Verification items for the finished model (mm, model axes). A direction names the side the tool comes from. Coordinates: 2 decimals unless noted, no trailing zeros. Write each loop counter-clockwise with the first axis right and the second up, starting at its lowest first coordinate (ties: lowest second). Pieces come first, ordered by that corner, then holes. Notation, with made-up numbers: M -9.75,23.25 L 36.25,23.25 A21 cw 36.25,41.25 Z; hole C 58.25,86.25 d6. An arc over 180 degrees is marked long. Answer in a Markdown table with one row per item.
Autodesk Inventor part; units mm, degrees
ref_plane "YZ Plane" through (0, 0, 0) normal (1, 0, 0) x (0, 1, 0)
ref_plane "XZ Plane" through (0, 0, 0) normal (0, 1, 0) x (-1, 0, 0)
ref_plane "XY Plane" through (0, 0, 0) normal (0, 0, 1) x (1, 0, 0)
sketch "Sketch1" plane through (0, 0, 0) normal (0, 1, 0) x (-1, 0, 0)
  line L0 (-25, 23) -> (25, 23)
  line L1 (25, 23) -> (25, -23)
  line L2 (25, -23) -> (-25, -23)
  line L3 (-25, -23) -> (-25, 23)
  line L4 (-25, 23) -> (25, -23) construction
  line L5 (25, 23) -> (-25, -23) construction
  circle A0 centre (12, 0) radius 4.15
  circle A1 centre (-15, -12) radius 2.65
  line L6 (25, 0) -> (-25, 0) construction
  circle A2 centre (-15, 12) radius 2.65
  point P0 (0, 0)
  dimension "d0" = 46
  dimension "d1" = 50
  dimension "d2" = 23
  dimension "d3" = 13
  dimension "d4" = 8.3
  dimension "d5" = 11
  dimension "d6" = 10
  dimension "d7" = 5.3
extrude "Extrusion1" add sketch "Sketch1" along normal blind 8
sketch "Sketch2" plane through (0, 0, 0) normal (0, -1, 0) x (1, 0, 0)
  line L0 (25, -23) -> (-25, -23)
  line L1 (25, 23) -> (25, -23)
  line L2 (-25, 23) -> (25, 23)
  line L3 (-25, -23) -> (-25, 23)
  circle A0 centre (15, 12) radius 2.65 construction
  circle A1 centre (15, -12) radius 2.65 construction
  circle A2 centre (-12, 0) radius 4.15
  circle A3 centre (15, -12) radius 2.65 construction
  circle A4 centre (15, -12) radius 5
  circle A5 centre (15, 12) radius 5
  point P0 (0, 0)
  dimension "d10" = 10
  dimension "d11" = 10
extrude "Extrusion2" cut sketch "Sketch2" against normal blind 5 contours A4 | A5
sketch "Sketch3" plane through (0, 8, 0) normal (0, 1, 0) x (1, 0, 0)
  circle A0 centre (13.5, 18.5) radius 3.15
  line L0 (25, -23) -> (25, 23)
  line L1 (25, 0) -> (-25, 0) construction
  line L2 (-25, 23) -> (-25, -23)
  line L3 (25, 23) -> (-25, 23)
  circle A1 centre (13.5, -18.5) radius 3.15
  point P0 (0, 0)
  dimension "d14" = 4.5
  dimension "d15" = 11.5
  dimension "d16" = 6.3
extrude "Extrusion3" cut sketch "Sketch3" against normal blind 3
sketch "Sketch5" plane through (0, 0, 0) normal (0, -1, 0) x (1, 0, 0)
  circle A0 centre (-12, 0) radius 4.15
  point P0 (0, 0)
extrude "Extrusion5" add sketch "Sketch5" against normal blind 1
equation "\"d11\" = d10"
properties part number "Linear Rail End Cap"
1) Sectioned sample at B-B (y = 7). Record the cut outline in (x, z), then the cut area to 3 significant figures.
Response values:
| item | result |
|---|---|
| outline | M -25,-23 L 25,-23 L 25,23 L -25,23 Z; hole C -12,0 d8.3; hole C 13.5,-18.5 d6.3; hole C 13.5,18.5 d6.3; hole C 15,-12 d5.3; hole C 15,12 d5.3 |
| area | 2,140 mm² |
2) Sectioned sample at C-C (x = 19). Record the cut outline in (y, z).
Response values:
| item | result |
|---|---|
| outline | M 0,-23 L 8,-23 L 8,23 L 0,23 L 0,15 L 5,15 L 5,9 L 0,9 L 0,-9 L 5,-9 L 5,-15 L 0,-15 Z |
3) Depth check by flat-ended pin: pin 1 (4 mm diameter, centred on x = 15, z = -12, fed in from -Y); pin 2 (6.5 mm diameter, centred on x = -12.5, z = 0, fed in from +Y); pin 3 (5 mm diameter, centred on x = 13.5, z = -11, fed in from -Y); pin 4 (5.5 mm diameter, centred on x = 13.5, z = 18.5, fed in from +Y). Enter the tip coordinate at first touch or a pass-through.
Response values:
| item | result |
|---|---|
| pin 1 | passes through |
| pin 2 | stops at y = 1 |
| pin 3 | stops at y = 5 |
| pin 4 | stops at y = 5 |
4) Release check for a two-part mould opening along X. For faces 1 (the face through (19.77, 2.46, 13.5)), 2 (the face through (0, 4, 23)), 3 (the face through (-25, 4, 0)), 4 (the face through (10.353, 6.521, 18.362)) record: +X half, -X half, draft (parallel to the pull), parting line (faces both ways), or undercut.
Response values:
| item | result |
|---|---|
| face 1 | undercut |
| face 2 | draft |
| face 3 | -X half |
| face 4 | undercut |
5) Sectioned sample at D-D (z = -12). Record the cut outline in (x, y).
Response values:
| item | result |
|---|---|
| outline | M -25,0 L 10,0 L 10,5 L 12.35,5 L 12.35,8 L -25,8 Z; M 17.65,5 L 20,5 L 20,0 L 25,0 L 25,8 L 17.65,8 Z |
6) Sectioned sample at A-A (y = 2). Record the cut outline in (x, z).
Response values:
| item | result |
|---|---|
| outline | M -25,-23 L 25,-23 L 25,23 L -25,23 Z; hole C -12,0 d8.3; hole C 15,-12 d10; hole C 15,12 d10 |
7) Thickness scan on L1, parallel to Z at x = 15, y = 2.7; L2, parallel to X at y = 7, z = -18.5; L3, parallel to X at y = 5.75, z = 0. Record the ranges inside material, lowest first. Write a range as [from, to].
Response values:
| item | result |
|---|---|
| L1 | z = [-23, -17], [-7, 7], [17, 23] |
| L2 | x = [-25, 10.35], [16.65, 25] |
| L3 | x = [-25, -16.15], [-7.85, 25] |
8) Tool access check on faces 5 (the face through (0, 4, -23)), 6 (the face through (17, 5, -10)), 7 (the face through (-12, 1, 0)). Record the directions out of +Z, -Z, +X, -X, +Y, -Y that give a thin tool (end or side, any length) a straight path to the whole face; none if there is none.
Response values:
| item | result |
|---|---|
| face 5 | -Z, +X, -X, +Y, -Y |
| face 6 | -Y |
| face 7 | +Y |
